Design review of the part shown in the three views and the two pictorial views. Dimensions are in mm from the part's minimum x, y and z. Give positions to 0.01 mm unless a question says otherwise; leave off trailing zeros. Order: outer loops, then holes, each group sorted by start corner. A loop starts at its lowest first (then second) coordinate and runs counter-clockwise, first axis right, second up. Notation, with made-up numbers: M 12,-6 L 70,-6 A22 ccw 70,16 Z; hole C 11.25,20.25 d9. An arc over 180 degrees is marked long. Answer as a JSON object with one key per item and string values.
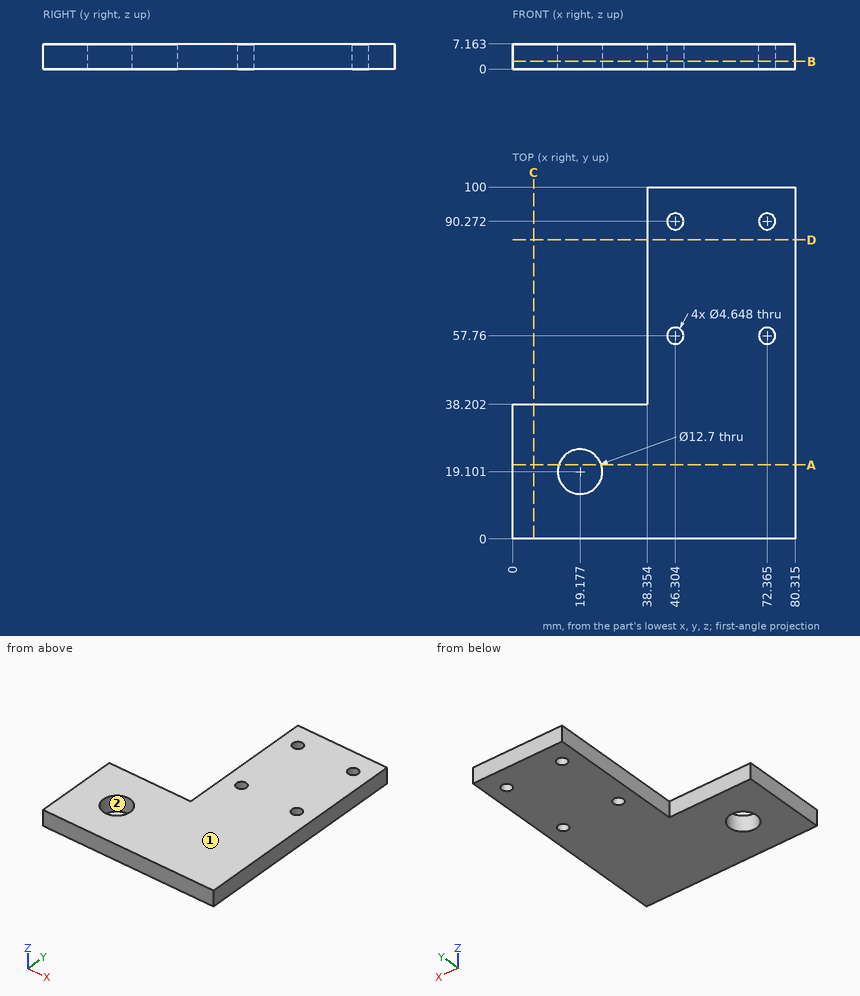
(1) Draft analysis for pull direction Y (two halves, no side actions). For the marked faces 1 and 2, state which applies: +Y half, -Y half, draft (parallel to the pull), parting line (faces both ways), or undercut.
Checked values:
{"face 1": "draft", "face 2": "undercut"}
(2) To check wall thickness, follow L1, parallel to X at y = 58.5, z = 2.5 (1 decimal); L2, parallel to X at y = 94.5, z = 6.25 (1 decimal); L3, parallel to Y at x = 37, z = 1. State the ranges of each line that lie inside material, in increasing order. Write a range as from..to.
Checked values:
{"L1": "x = 38.4..44.1, 48.5..70.2, 74.6..80.3", "L2": "x = 38.4..80.3", "L3": "y = 0..38.2"}
(3) We need section B-B (z = 2.25). Count the separate pieces of the cut face and the enclosed holes in it, plus the area to 3 significant figures.
Checked values:
{"separate pieces": "1", "enclosed holes": "5", "area": "5,470 mm^2"}
(4) We need section D-D (y = 85). Write out the cut boundary in (x, z) (1 decimal).
Checked values:
{"outline": "M 38.4,0 L 80.3,0 L 80.3,7.2 L 38.4,7.2 Z"}
(5) We need section A-A (y = 21). Write out the cut boundary in (x, z) (1 decimal).
Checked values:
{"outline": "M 0,0 L 13.1,0 L 13.1,7.2 L 0,7.2 Z; M 25.2,0 L 80.3,0 L 80.3,7.2 L 25.2,7.2 Z"}
(6) We need section C-C (x = 6). Write out the cut boundary in (y, z).
Checked values:
{"outline": "M 0,0 L 38.2,0 L 38.2,7.16 L 0,7.16 Z"}
(7) Insertion check: pin 1 (4 mm diameter, centred on x = 72.36, y = 90.27, fed in from -Z); pin 2 (1.5 mm diameter, centred on x = 16, z = 2, fed in from +Y). Each pin has a flat end and moves straight along its axis. Give the tip position at first contact, or say it passes through.
Checked values:
{"pin 1": "passes through", "pin 2": "stops at y = 38.2"}
